Build history of the part. All positions in model axes, mm. A direction names the side the tool comes from. Give positions to 0.01 mm unless a question says otherwise; leave off trailing zeros. Write each loop counter-clockwise with the first axis right and the second up, starting at its lowest first coordinate (ties: lowest second). Pieces come first, ordered by that corner, then holes. Notation, with made-up numbers: (-1, 0.25) -> (47, 0.25) arc R25 ccw to (47, 21.25) -> close; hole circle Ø8 at (42, 83). An arc over 180 degrees is marked (long way). Write item = value, one per line. Start each with the question number.
Q1. Saw through at B-B, the plane z = 5.5. List the corners of the cut face in (x, y).
Q2. Mould opens along X. For faces 6 (the face through (0, 15, 2)), 7 (the face through (10.637, 15.535, -1.821)), 8 (the face through (-0.6, 18, -3)), 9 (the face through (4, 10, 4)) say: pulls with the +X half, pulls with the -X half, needs draft (parallel to the pull), parting line crosses it, or undercut.
Q3. Saw through at D-D, the plane y = 14. List the corners of the cut face in (x, z) (3 decimals), then the cut area to 3 significant figures.
Q4. Tool access for faces 1 (the face through (-10, 13, -1)), 2 (the face through (6, 10, 2.026)), 3 (the face through (0.6, 18, -3)), 4 (the face through (0, 14, 0)), 5 (the face through (-10, 18, 2.026)): list every direction of +Z, -Z, +X, -X, +Y, -Y with a clear straight run to the whole face (end or side of a thin tool).
Q5. Wall check: line 1 (Z direction, x = 1.25, y = 20); line 2 (Z direction, x = 12, y = 14.1) (3 decimals); line 3 (X direction, y = 14.5, z = -1). Give the ranges that are in metal, low to high.
Q6. Drop flat-ended pins along their axis: P1, Ø3, axis at x = 12, z = -2, coming from the -Y side; P2, Ø2.5, axis at x = -12, z = -2, coming from the -Y side; P3, Ø1.6, axis at y = 10.5, z = 3.5, coming from the +X side. Give the stop position or say it passes through.
Q7. Saw through at A-A, the plane x = 0. List the corners of the cut face in (y, z).
Q8. Saw through at C-C, the plane y = 21. List the corners of the cut face in (x, z), then the cut area to 3 significant figures.
Autodesk Fusion 360 part; units mm, degrees
sketch "スケッチ1" plane through (0, 0, 0) normal (0, 0, 1) x (1, 0, 0)
  line L0 (-16.5, 22) -> (16.5, 22)
  line L1 (16.5, 22) -> (16.5, 0)
  line L2 (16.5, 0) -> (-16.5, 0)
  line L3 (-16.5, 0) -> (-16.5, 22)
  dimension "d7" = 22
  dimension "d8" = 33
extrude "押し出し1" add sketch "スケッチ1" along normal blind 2
sketch "スケッチ3" plane through (0, 0, 0) normal (0, 0, -1) x (1, 0, 0)
  line L0 (16.5, 0) -> (-16.5, 0)
  line L1 (-16.5, 0) -> (-16.5, -22)
  line L2 (-16.5, -22) -> (16.5, -22)
  line L3 (16.5, -22) -> (16.5, 0)
  arc A0 (-8.9, -13) -> (8.9, -13) centre (0, -13) ccw
  line L4 (16.5, -13) -> (-16.5, -13)
  dimension "d9" = 17.8
  dimension "d10" = 9
extrude "押し出し2" add sketch "スケッチ3" along normal blind 2 contours L1 L2 L3 A0 L4
sketch "スケッチ4" plane through (0, 0, -2) normal (0, 0, -1) x (1, 0, 0)
  line L0 (-8.9, -13) -> (-16.5, -13)
  line L1 (-16.5, -13) -> (-16.5, -22)
  line L2 (-16.5, -22) -> (16.5, -22)
  line L3 (16.5, -22) -> (16.5, -13)
  line L4 (16.5, -13) -> (8.9, -13)
  arc A0 (-8.9, -13) -> (8.9, -13) centre (0, -13) ccw
  line L5 (16.5, -22) -> (0.6, -22)
  line L6 (0.6, -22) -> (0.6, -13)
  line L7 (0.6, -13) -> (16.5, -13)
  line L8 (16.5, -13) -> (16.5, -22)
  line L9 (-16.5, -22) -> (-0.6, -22)
  line L10 (-0.6, -22) -> (-0.6, -13)
  line L11 (-0.6, -13) -> (-16.5, -13)
  line L12 (-16.5, -13) -> (-16.5, -22)
  dimension "d13" = 1.2
extrude "押し出し3" add sketch "スケッチ4" along normal blind 2
sketch "スケッチ5" plane through (0, 0, 0) normal (0, 0, -1) x (1, 0, 0)
  line L0 (8.9, -13) -> (16.5, -13)
  line L1 (16.5, -13) -> (16.5, 0)
  line L2 (16.5, 0) -> (-16.5, 0)
  line L3 (-16.5, 0) -> (-16.5, -13)
  line L4 (-16.5, -13) -> (-8.9, -13)
  arc A0 (-8.9, -13) -> (8.9, -13) centre (0, -13) ccw
  line L5 (-3.75, 0) -> (3.75, 0)
  line L6 (3.75, 0) -> (3.75, -18)
  line L7 (3.75, -18) -> (-3.75, -18)
  line L8 (-3.75, -18) -> (-3.75, 0)
  line L9 (0, -1.75) -> (0, -22.5)
  line L10 (3.75, -7) -> (16.5, -7)
  line L11 (-3.75, -7) -> (-16.5, -7)
  dimension "d17" = 7.5
  dimension "d18" = 11
  dimension "d19" = 11
sketch "スケッチ9" plane through (0, 13, 0) normal (0, -1, 0) x (1, 0, 0)
  line L0 (-8.9, 0) -> (-16.5, 0)
  line L1 (-16.5, 0) -> (-16.5, -4)
  line L2 (-16.5, -4) -> (-0.6, -4)
  line L3 (-0.6, -4) -> (-0.6, -2)
  line L4 (-0.6, -2) -> (-8.9, -2)
  line L5 (-8.9, -2) -> (-8.9, 0)
  line L6 (-5.25, -2) -> (5.25, -2)
  line L7 (5.25, -2) -> (5.25, -4)
  line L8 (5.25, -4) -> (-5.25, -4)
  line L9 (-5.25, -4) -> (-5.25, -2)
  line L10 (16.5, -4) -> (0.6, -4)
  dimension "d37" = 10.5
  dimension "d38" = 5.25
extrude "押し出し7" cut sketch "スケッチ9" against normal blind 1.5 contours L2 L3 L4 L6 L8 L9 | L3 L6 L7 L8 L10
sketch "スケッチ11" plane through (0, 22, 0) normal (0, 1, 0) x (-1, 0, 0)
  line L0 (16.5, -4) -> (16.5, 2)
  line L1 (16.5, 2) -> (-16.5, 2)
  line L2 (-16.5, 2) -> (-16.5, -4)
  line L3 (-16.5, -4) -> (16.5, -4)
  line L4 (16.5, 2) -> (-13.5, 2)
  line L5 (-13.5, 2) -> (-13.5, 12)
  line L6 (-13.5, 12) -> (16.5, 12)
  line L7 (16.5, 12) -> (16.5, 2)
  dimension "d49" = 10
ref_plane "作業平面1" through (0, 11, -1) normal (0, 1, 0) x (-1, 0, 0)
sketch "スケッチ13" plane through (0, 11, -1) normal (0, 1, 0) x (1, 0, 0)
  line L0 (16.5, -10) -> (-16.5, -10)
  line L1 (-16.5, -10) -> (-16.5, -3)
  line L2 (-16.5, -3) -> (16.5, -3)
  line L3 (16.5, -3) -> (16.5, -10)
  line L4 (16.5, 3) -> (16.5, -3)
  line L5 (-16.5, 3) -> (-16.5, -3)
  circle A0 centre (0, -6.5) radius 2.25
  dimension "d53" = 7
  dimension "d54" = 4.5
  dimension "d58" = 3.5
extrude "押し出し11" add sketch "スケッチ13" along normal blind -2 and the other way blind -8
sketch "Sketch17" plane through (16.5, 0, 0) normal (1, 0, 0) x (0, 1, 0)
  line L0 (22, -4) -> (22, 2)
  line L1 (22, 2) -> (19, 2)
  line L2 (19, 2) -> (19, 9)
  line L3 (19, 9) -> (9, 9)
  line L4 (9, 9) -> (9, 2)
  line L5 (9, 2) -> (0, 2)
  line L6 (0, 2) -> (0, 0)
  line L7 (0, 0) -> (13, 0)
  line L8 (13, 0) -> (13, -4)
  line L9 (13, -4) -> (22, -4)
  line L10 (11, 9) -> (17, 9)
  line L11 (17, 9) -> (17, 2)
  line L12 (17, 2) -> (11, 2)
  line L13 (11, 2) -> (11, 9)
extrude "Extrude15" cut sketch "Sketch17" against normal blind 400 contours L3 L10 L11 L12 L13
sketch "Sketch18" plane through (-16.5, 0, 0) normal (-1, 0, 0) x (0, -1, 0)
  line L0 (-11, 9) -> (-11, 2)
  line L1 (-11, 2) -> (-17, 2)
  line L2 (-17, 2) -> (-17, 9)
  line L3 (-17, 9) -> (-19, 9)
  line L4 (-19, 9) -> (-19, 2)
  line L5 (-19, 2) -> (-22, 2)
  line L6 (-22, 2) -> (-22, -4)
  line L7 (-22, -4) -> (-13, -4)
  line L8 (-13, -4) -> (-13, 0)
  line L9 (-13, 0) -> (0, 0)
  line L10 (0, 0) -> (0, 2)
  line L11 (0, 2) -> (-9, 2)
  line L12 (-9, 2) -> (-9, 9)
  line L13 (-9, 9) -> (-11, 9)
  line L14 (-9, 2) -> (0, 2)
  line L15 (0, 2) -> (0, 0)
  line L16 (0, 0) -> (-9, 0)
  line L17 (-9, 0) -> (-9, 2)
extrude "Extrude16" cut sketch "Sketch18" against normal blind 34 contours L9 L10 L11 L14 L15 L16 L17
sketch "Sketch19" plane through (0, 13, 0) normal (0, -1, 0) x (1, 0, 0)
  line L0 (5.25, -2) -> (5.25, -4)
  line L1 (5.25, -4) -> (16.5, -4)
  line L2 (16.5, -4) -> (16.5, 0)
  line L3 (16.5, 0) -> (8.9, 0)
  line L4 (8.9, 0) -> (8.9, -2)
  line L5 (8.9, -2) -> (5.25, -2)
  line L6 (0.6, -2) -> (16.5, -2)
  line L7 (-0.6, -2) -> (-16.5, -2)
  point P0 (12, -2)
  point P1 (-12, -2)
hole "Hole1" at (-12, 13, -2) at (12, 13, -2) direction (0, 1, 0) diameter 2.75 depth 5 tip angle 118
sketch "Sketch20" plane through (0, 9, 0) normal (0, -1, 0) x (1, 0, 0)
  circle A0 centre (0, 5.5) radius 2.25
  line L0 (16.5, 0) -> (16.5, 9)
  line L1 (16.5, 9) -> (-16.5, 9)
  line L2 (-16.5, 9) -> (-16.5, 0)
  line L3 (-16.5, 0) -> (16.5, 0)
  circle A1 centre (0, 5) radius 4
  curve L4
  curve L5
  curve L6
  curve L7
  line L8 (-16.5, 2.0263) -> (16.5, 2.0263)
  line L9 (16.5, 2.0263) -> (16.5, 0)
  line L10 (16.5, 0) -> (-16.5, 0)
  line L11 (-16.5, 0) -> (-16.5, 2.0263)
  line L12 (-4, 5) -> (-4, 2.0263)
  line L13 (4, 5) -> (4, 2.0263)
  point P0 (-16.5, 2)
extrude "Extrude17" cut sketch "Sketch20" against normal blind 150 contours L0 L1 A1 L8 L13 | L1 L2 A1 L8 L12
sketch "Sketch21" plane through (0, 0, -4) normal (0, 0, -1) x (1, 0, 0)
  line L0 (5.25, -13) -> (5.25, -14.5)
  line L1 (5.25, -14.5) -> (0.6, -14.5)
  line L2 (0.6, -14.5) -> (0.6, -21.8798)
  arc A0 (-0.6, -21.8798) -> (0.6, -21.8798) centre (0, -13) ccw
  line L3 (-0.6, -21.8798) -> (-0.6, -14.5)
  line L4 (-0.6, -14.5) -> (-5.25, -14.5)
  line L5 (-5.25, -14.5) -> (-5.25, -13)
  line L6 (-5.25, -13) -> (-16.5, -13)
  line L7 (-16.5, -13) -> (-16.5, -22)
  line L8 (-16.5, -22) -> (16.5, -22)
  line L9 (16.5, -22) -> (16.5, -13)
  line L10 (16.5, -13) -> (5.25, -13)
sketch "Sketch22" plane through (0, 0, 0) normal (0, 0, -1) x (1, 0, 0)
  line L0 (16.5, -9) -> (-16.5, -9)
  line L1 (-16.5, -9) -> (-16.5, -13)
  line L2 (-16.5, -13) -> (-8.9, -13)
  arc A0 (-8.9, -13) -> (8.9, -13) centre (0, -13) ccw
  line L3 (8.9, -13) -> (16.5, -13)
  line L4 (16.5, -13) -> (16.5, -9)
  circle A1 centre (0, -13) radius 9
extrude "Extrude18" cut sketch "Sketch22" against normal blind 10 contours L0 L3 L4 A1 | L0 L1 L2 A1
move_face "OffsetFaces1" offset -1 1 faces at (16.5, 17.3333, -2)
move_face "OffsetFaces2" offset -0.5 1 faces at (15.5, 17.3333, -2)
move_face "OffsetFaces3" offset -1.5 1 faces at (-16.5, 17.3333, -2)
move_face "OffsetFaces4" offset 1 1 faces at (5, 22, 0)
move_face "OffsetFaces5" offset -1 1 faces at (5, 23, 0)
Report:
q1.outline = (-3.97, 9) -> (-2.25, 9) -> (-2.25, 11) -> (-3.97, 11) -> close; (-3.97, 17) -> (-2.25, 17) -> (-2.25, 19) -> (-3.97, 19) -> close; (2.25, 9) -> (3.97, 9) -> (3.97, 11) -> (2.25, 11) -> close; (2.25, 17) -> (3.97, 17) -> (3.97, 19) -> (2.25, 19) -> close
q2.face_6 = needs draft
q2.face_7 = undercut
q2.face_8 = undercut
q2.face_9 = pulls with the +X half
q3.outline = (-15, -4) -> (-5.25, -4) -> (-5.25, -2) -> (-8.844, -2) -> (-8.844, 0) -> (8.844, 0) -> (8.844, -2) -> (5.25, -2) -> (5.25, -4) -> (15, -4) -> (15, 2) -> (-15, 2) -> close; hole circle Ø2.75 at (-12, -2); hole circle Ø2.75 at (12, -2)
q3.area = 112 mm2
q4.face_1 = -Z, -X, -Y
q4.face_2 = +Z, +X, +Y, -Y
q4.face_3 = -Z, -Y
q4.face_4 = -Y
q4.face_5 = +Z, -X, +Y, -Y
q5.line_1 = -4 to -2, 0 to 2
q5.line_2 = -4 to -3.375, -0.625 to 2
q5.line_3 = -15 to -12.94, -11.06 to -8.77, 8.77 to 11.06, 12.94 to 15
q6.P1 = 13
q6.P2 = 18.08
q6.P3 = 4
q7.outline = (9, 0) -> (21.9, 0) -> (21.9, -4) -> (22, -4) -> (22, 2) -> (19, 2) -> (19, 3.25) -> (17, 3.25) -> (17, 2) -> (11, 2) -> (11, 3.25) -> (9, 3.25) -> close; (9, 7.75) -> (11, 7.75) -> (11, 9) -> (9, 9) -> close; (17, 7.75) -> (19, 7.75) -> (19, 9) -> (17, 9) -> close
q8.outline = (-15, -4) -> (-0.6, -4) -> (-0.6, -2) -> (-3.9, -2) -> (-3.9, 0) -> (3.9, 0) -> (3.9, -2) -> (0.6, -2) -> (0.6, -4) -> (15, -4) -> (15, 2) -> (-15, 2) -> close
q8.area = 162 mm2
